Verification items for the finished model (mm, model axes). Face numbers are marked on the shaded views. A direction names the side the tool comes from. Coordinates: 2 decimals unless noted, no trailing zeros. Order: outer loops, then holes, each group sorted by start corner. A loop starts at its lowest first (then second) coordinate and runs counter-clockwise, first axis right, second up. Notation, with made-up numbers: M 11.25,50.25 L 42.25,50.25 A19 ccw 42.25,59.25 Z; hole C -13.5,37 d5. An arc over 180 degrees is marked long. Answer as a JSON object with one key per item and string values. Group by question number.
(1) Access from +Z, -Z, +X, -X, +Y, -Y to the whole of each face (thin tool, end or side, straight path). Record for the marked faces 1, 2 and 3.
(2) Cross-section at C-C (z = 16). Enter the section's corners in (x, y) (3 decimals), plus the area to 3 significant figures.
(3) Material ranges on line 1 (Z direction, x = 19.05, y = 11.25); line 2 (Z direction, x = 36.5, y = 28); line 3 (Z direction, x = 19.5, y = 12), recorded low to high.
(4) Cross-section at B-B (x = 29.55). Enter the section's corners in (y, z), plus the area to 3 significant figures.
(5) Cross-section at A-A (y = 46.5). Enter the section's corners in (x, z), plus the area to 3 significant figures.
(6) Cross-section at D-D (y = 9). Enter the section's corners in (x, z).
(7) Gauge pin test, flat ends, axial feed: pin 1 Ø10 at (x, z) = (22.5, 28.5) entering from +Y; pin 2 Ø5 at (x, z) = (11.5, 6) entering from +Y; pin 3 Ø5.5 at (x, z) = (19.05, 23.02) entering from +Y. Record the tip position at first contact, or that the pin passes through.
(8) Mould release check, pull along X, two halves, no side actions. Record for the marked faces 4, 5 and 6: released by +X, released by -X, zero draft, split by the parting line, or undercut.
from build123d import *

# Parameters (mm, degrees)
BOSS_EXTRUDE1_DEPTH = 46.0375
FILLET1_R           = 3.175
CUT_EXTRUDE1_DEPTH  = 16.66875
SKETCH3_R           = 0.999998
SKETCH3_R_2         = 1.75
CUT_EXTRUDE2_DEPTH  = 6.35
SKETCH4_R           = 3.96875
CUT_EXTRUDE3_DEPTH  = 6.35
CUT_EXTRUDE4_DEPTH  = 3
SKETCH6_R           = 1.75
SKETCH6_R_2         = 1
CUT_EXTRUDE5_DEPTH  = 9.7
SKETCH7_R           = 3
CUT_EXTRUDE6_DEPTH  = 6.35
SKETCH9_R           = 0.999998
SKETCH9_R_2         = 1.75
CUT_EXTRUDE7_DEPTH  = 3


with BuildPart() as part:
    # Sketch1 → Boss-Extrude1 (new body)
    with BuildSketch(Plane.XY):
        with BuildLine():
            Line((0, 0), (38.1, 0))
            Line((38.1, 0), (38.1, 31.75))
            ThreePointArc((38.1, 31.75), (19.05, 50.8), (0, 31.75))
            Line((0, 31.75), (0, 0))
        make_face()
    extrude(amount=BOSS_EXTRUDE1_DEPTH)

    # Fillet1
    fillet1_edges = [part.edges().sort_by_distance(p)[0] for p in [
        (38.1, 0, 23.01875),
        (0, 0, 23.01875),
    ]]
    fillet(fillet1_edges, radius=FILLET1_R)

    # Sketch2 → Cut-Extrude1 (cut, symmetric)
    with BuildSketch(Plane(origin=(0, 0, 23.01875), x_dir=(-1, 0, 0), z_dir=(0, 0, -1))):
        with BuildLine():
            Line((-38.1, 31.75), (-38.1, 12.7))
            Line((-38.1, 12.7), (0, 12.7))
            Line((0, 12.7), (0, 31.75))
            ThreePointArc((0, 31.75), (-19.05, 50.8), (-38.1, 31.75))
        make_face()
    extrude(amount=CUT_EXTRUDE1_DEPTH, both=True, mode=Mode.SUBTRACT)

    # Sketch3 → Cut-Extrude2 (cut)
    with BuildSketch(Plane.XY.offset(6.35)):
        with Locations((8.55, 38.1)):
            Circle(SKETCH3_R)
        with Locations((29.55, 38.1)):
            Circle(SKETCH3_R)
        with Locations((19.05, 38.1)):
            Circle(SKETCH3_R_2)
    extrude(amount=-CUT_EXTRUDE2_DEPTH, mode=Mode.SUBTRACT)

    # Sketch4 → Cut-Extrude3 (cut)
    with BuildSketch(Plane(origin=(0, 0, 39.6875), x_dir=(-1, 0, 0), z_dir=(0, 0, -1))):
        with Locations((-19.05, 38.1)):
            Circle(SKETCH4_R)
    extrude(amount=-CUT_EXTRUDE3_DEPTH, mode=Mode.SUBTRACT)

    # Sketch5 → Cut-Extrude4 (cut)
    with BuildSketch(Plane.XZ):
        with BuildLine():
            Line((23.266666152, 22.4875), (21.530391854, 8.70625))
            ThreePointArc((21.530391854, 8.70625), (19.05, 6.51875), (16.569608146, 8.70625))
            Line((16.569608146, 8.70625), (14.833333848, 22.4875))
            ThreePointArc((14.833333848, 22.4875), (14.8, 23.01875), (14.833333848, 23.55))
            Line((14.833333848, 23.55), (16.569608146, 37.33125))
            ThreePointArc((16.569608146, 37.33125), (19.05, 39.51875), (21.530391854, 37.33125))
            Line((21.530391854, 37.33125), (23.266666152, 23.55))
            ThreePointArc((23.266666152, 23.55), (23.3, 23.01875), (23.266666152, 22.4875))
        make_face()
    extrude(amount=-CUT_EXTRUDE4_DEPTH, mode=Mode.SUBTRACT)

    # Sketch6 → Cut-Extrude5 (cut)
    with BuildSketch(Plane.XZ.offset(-3)):
        with Locations((19.05, 23.01875)):
            Circle(SKETCH6_R)
        with Locations((19.05, 33.51875)):
            Circle(SKETCH6_R_2)
        with Locations((19.05, 12.51875)):
            Circle(SKETCH6_R_2)
    extrude(amount=-CUT_EXTRUDE5_DEPTH, mode=Mode.SUBTRACT)

    # Sketch7 → Cut-Extrude6 (cut)
    with BuildSketch(Plane(origin=(0, 12.7, 0), x_dir=(1, 0, 0), z_dir=(0, 1, 0))):
        with Locations((19.05, -23.01875)):
            Circle(SKETCH7_R)
    extrude(amount=-CUT_EXTRUDE6_DEPTH, mode=Mode.SUBTRACT)

    # Sketch9 → Cut-Extrude7 (cut)
    with BuildSketch(Plane.XY.offset(6.35)):
        with BuildLine():
            Line((4.248275862, 40.581725719), (18.537068966, 42.318933722))
            ThreePointArc((18.537068966, 42.318933722), (19.05, 42.35), (19.562931034, 42.318933722))
            Line((19.562931034, 42.318933722), (33.851724138, 40.581725719))
            ThreePointArc((33.851724138, 40.581725719), (36.05, 38.1), (33.851724138, 35.618274281))
            Line((33.851724138, 35.618274281), (19.562931034, 33.881066278))
            ThreePointArc((19.562931034, 33.881066278), (19.05, 33.85), (18.537068966, 33.881066278))
            Line((18.537068966, 33.881066278), (4.248275862, 35.618274281))
            ThreePointArc((4.248275862, 35.618274281), (2.05, 38.1), (4.248275862, 40.581725719))
        make_face()
        with Locations((8.55, 38.1)):
            Circle(SKETCH9_R, mode=Mode.SUBTRACT)
        with Locations((29.55, 38.1)):
            Circle(SKETCH9_R, mode=Mode.SUBTRACT)
        with Locations((19.05, 38.1)):
            Circle(SKETCH9_R_2, mode=Mode.SUBTRACT)
    extrude(amount=-CUT_EXTRUDE7_DEPTH, mode=Mode.SUBTRACT)


solid = part.part
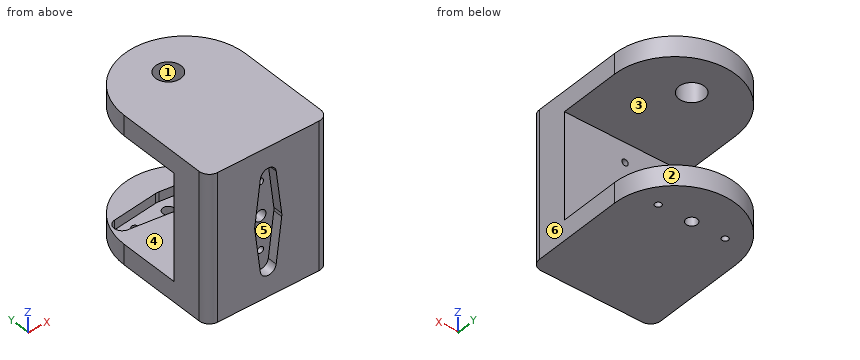
Taken from the geometry:
{
 "1": {"face 1": "+Z", "face 2": "+Z, -Z, +Y", "face 3": "+X, -X, +Y"},
 "2": {"outline": "M 0,3.175 A3.175 ccw 3.175,0 L 15.651,0 L 15.651,3 L 22.449,3 L 22.449,0 L 34.925,0 A3.175 ccw 38.1,3.175 L 38.1,12.7 L 0,12.7 Z", "area": "459 mm²"},
 "3": {"line 1": "z = 0 to 11.52, 13.52 to 20.02, 26.02 to 32.52, 34.52 to 46.04", "line 2": "z = 0 to 6.35, 39.69 to 46.04", "line 3": "z = 0 to 11.63, 13.41 to 20.05, 25.98 to 32.63, 34.41 to 46.04"},
 "4": {"outline": "M 0,0 L 37.1,0 L 37.1,3.35 L 35.1,3.35 L 35.1,6.35 L 12.7,6.35 L 12.7,39.69 L 47.65,39.69 L 47.65,46.04 L 0,46.04 Z; M 39.1,0 L 47.65,0 L 47.65,6.35 L 41.1,6.35 L 41.1,3.35 L 39.1,3.35 Z", "area": "1,000 mm²"},
 "5": {"outline": "M 6.99,0 L 31.11,0 L 31.11,6.35 L 6.99,6.35 Z; M 6.99,39.69 L 31.11,39.69 L 31.11,46.04 L 6.99,46.04 Z", "area": "306 mm²"},
 "6": {"outline": "M 0,0 L 38.1,0 L 38.1,46.04 L 0,46.04 Z; hole C 19.05,23.02 d6; hole C 19.05,12.52 d2; hole C 19.05,33.52 d2"},
 "7": {"pin 1": "stops at y = 12.7", "pin 2": "stops at y = 50.12", "pin 3": "stops at y = 6.35"},
 "8": {"face 4": "zero draft", "face 5": "undercut", "face 6": "released by +X"}
}
